Check sheet for the modelled part. Datum: model origin and axes. Units: mm. Face numbers are marked on the shaded views. Round coordinates to 2 decimals unless told otherwise and drop trailing zeros. Write each loop counter-clockwise with the first axis right and the second up, starting at its lowest first coordinate (ties: lowest second). Pieces come first, ordered by that corner, then holes. Notation, with made-up numbers: M 87.25,72.25 L 139.25,72.25 A15 cw 139.25,99.25 Z; hole C 63.25,-26 d11. An arc over 180 degrees is marked long. Answer in a Markdown table with one row per item.
```python
from build123d import *

# Parameters (mm, degrees)
ESQUISSE1_W             = 27
ESQUISSE1_H             = 11.300000191
BOSS_EXTRU_1_DEPTH      = 5
ENL_V_MAT_EXTRU_1_DEPTH = 30.693265302
ENL_V_MAT_EXTRU_2_DEPTH = 30.693265302
ENL_V_MAT_EXTRU_3_DEPTH = 30.693265302
ENL_V_MAT_EXTRU_4_DEPTH = 30.693265302
D_POUILLE1_ANGLE        = 19.197649098
D_POUILLE2_ANGLE        = 19.197649098


with BuildPart() as part:
    # Esquisse1 → Boss.-Extru.1 (new body)
    with BuildSketch(Plane(origin=(0, 0, 0), x_dir=(-1, 0, 0), z_dir=(0, 0, -1))):
        with Locations((-13.5, 5.650000096)):
            Rectangle(ESQUISSE1_W, ESQUISSE1_H)
    extrude(amount=-BOSS_EXTRU_1_DEPTH)

    # Esquisse2 → Enlèv. mat.-Extru.1 (cut, through all)
    with BuildSketch(Plane(origin=(0, 11.300000191, 0), x_dir=(-1, 0, 0), z_dir=(0, 1, 0))):
        Polygon((-15.372982979, 5), (-15.372982979, 4.774707955), (-14.840999603, 3.800517559), (-14.434993744, 3.282314301), (-13.949490547, 2.83772254), (-13.397639275, 2.478783607), (-12.794389725, 2.21522069), (-12.156080246, 2.054171801), (-11.5, 2), (-10.843919754, 2.054171801), (-10.205610275, 2.21522069), (-9.602360725, 2.478783607), (-9.050509453, 2.83772254), (-8.56500721, 3.282314301), (-8.159000397, 3.800517559), (-7.627017021, 4.774707955), (-7.627017021, 5), align=None)
    extrude(amount=-ENL_V_MAT_EXTRU_1_DEPTH, mode=Mode.SUBTRACT)

    # Esquisse3 → Enlèv. mat.-Extru.2 (cut, through all)
    with BuildSketch(Plane(origin=(0, 11.300000191, 0), x_dir=(-1, 0, 0), z_dir=(0, 1, 0))):
        with BuildLine():
            Line((-20.75, 5), (-24.25, 5))
            ThreePointArc((-24.25, 5), (-22.5, 3.25), (-20.75, 5))
        make_face()
    extrude(amount=-ENL_V_MAT_EXTRU_2_DEPTH, mode=Mode.SUBTRACT)

    # Esquisse4 → Enlèv. mat.-Extru.3 (cut, through all)
    with BuildSketch(Plane(origin=(0, 0, 0), x_dir=(-1, 0, 0), z_dir=(0, 0, -1))):
        Polygon((-2.75, 5.650000095), (-2.775172234, 5.945751667), (-2.84996438, 6.232994556), (-2.972225189, 6.503466129), (-3.13843751, 6.74938488), (-3.343819141, 6.963676453), (-3.582462311, 7.140175819), (-3.847501278, 7.273805618), (-4.13131094, 7.360721588), (-4.425727844, 7.398423195), (-4.722281456, 7.385825634), (-5.012440205, 7.323291779), (-5.287856102, 7.212620258), (-5.540607929, 7.056994915), (-5.763422966, 6.86089325), (-5.949892044, 6.629955769), (-6.094649792, 6.370827198), (-6.193532467, 6.090961456), (-6.243695736, 5.798409939), (-6.25, 5.650000095), (-6.243695736, 5.501589775), (-6.193532467, 5.209038734), (-6.094649792, 4.929172993), (-5.949892044, 4.670043945), (-5.763422966, 4.439106941), (-5.540607929, 4.243005276), (-5.287856102, 4.087379456), (-5.012440205, 3.976708174), (-4.722281456, 3.91417408), (-4.425727844, 3.901576757), (-4.13131094, 3.939278364), (-3.847501278, 4.026194096), (-3.582462311, 4.159823895), (-3.343819141, 4.336323738), (-3.13843751, 4.550614834), (-2.972225189, 4.796534061), (-2.84996438, 5.067005157), (-2.775172234, 5.354248524), align=None)
    extrude(amount=-ENL_V_MAT_EXTRU_3_DEPTH, mode=Mode.SUBTRACT)

    # Esquisse5 → Enlèv. mat.-Extru.4 (cut, through all)
    with BuildSketch(Plane.XY.offset(5)):
        Polygon((16.77517128, 5.354248524), (16.849964142, 5.067005157), (16.972225189, 4.796534061), (17.138439178, 4.550614834), (17.343818665, 4.336323738), (17.582462311, 4.159823895), (17.847499847, 4.026194096), (18.131311417, 3.939278364), (18.425727844, 3.901576757), (18.722280502, 3.91417408), (19.012439728, 3.976708174), (19.287857056, 4.087379456), (19.540607452, 4.243005276), (19.76342392, 4.439106941), (19.949892044, 4.670043945), (20.094650269, 4.929172993), (20.193532944, 5.209038734), (20.243694305, 5.501589775), (20.243694305, 5.798409939), (20.193532944, 6.090961456), (20.094650269, 6.370827198), (19.949892044, 6.629955769), (19.76342392, 6.86089325), (19.540607452, 7.056994915), (19.287857056, 7.212620258), (19.012439728, 7.323291779), (18.722280502, 7.385825634), (18.425727844, 7.398423195), (18.131311417, 7.360721588), (17.847499847, 7.273805618), (17.582462311, 7.140175819), (17.343818665, 6.963676453), (17.138439178, 6.74938488), (16.972225189, 6.503466129), (16.849964142, 6.232994556), (16.77517128, 5.945751667), (16.75, 5.650000095), align=None)
    extrude(amount=-ENL_V_MAT_EXTRU_4_DEPTH, mode=Mode.SUBTRACT)

    # Dépouille1
    d_pouille1_faces = [part.faces().sort_by_distance(p)[0] for p in [
        (7.627017021, 5.650000095, 4.887353977),
    ]]
    draft(d_pouille1_faces, Plane.XY.offset(5), D_POUILLE1_ANGLE)

    # Dépouille2
    d_pouille2_faces = [part.faces().sort_by_distance(p)[0] for p in [
        (15.372982979, 5.650000095, 4.887353977),
    ]]
    draft(d_pouille2_faces, Plane.XY.offset(5), D_POUILLE2_ANGLE)


solid = part.part
```
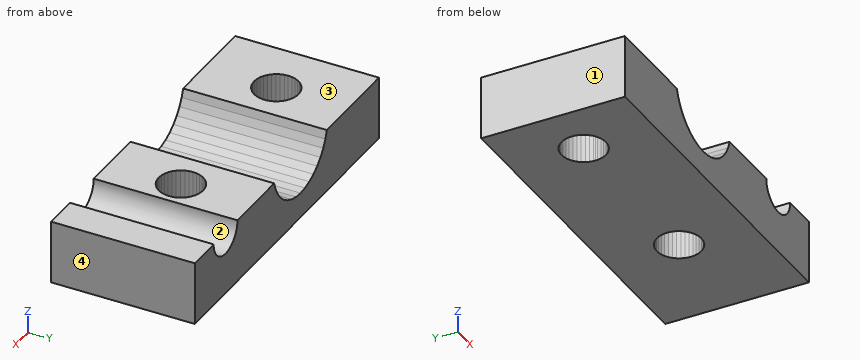
1. Draft check along X on the marked faces 1, 2, 3 and 4. Enter one of: +X half, -X half, draft (parallel to the pull), parting line (faces both ways), or undercut.
Found:
| item | result |
|---|---|
| face 1 | -X half |
| face 2 | undercut |
| face 3 | draft |
| face 4 | +X half |
2. Section check B-B, the plane x = 22.5. Record the cut outline in (y, z), and give its area (3 significant figures).
Found:
| item | result |
|---|---|
| outline | M 0,0 L 11.3,0 L 11.3,3.25 L 0,3.25 Z |
| area | 36.7 mm2 |
3. Scan lines: L1, parallel to Y at x = 18.75, z = 4.8; L2, parallel to X at y = 10, z = 3.6; L3, parallel to X at y = 3.75, z = 4.45. Record each from-to range of solid material in increasing order.
Found:
| item | result |
|---|---|
| L1 | y = 0 to 3.92, 7.38 to 11.3 |
| L2 | x = 0 to 8.32, 14.68 to 21.45, 23.55 to 27 |
| L3 | x = 0 to 7.82, 15.18 to 20.84, 24.16 to 27 |
